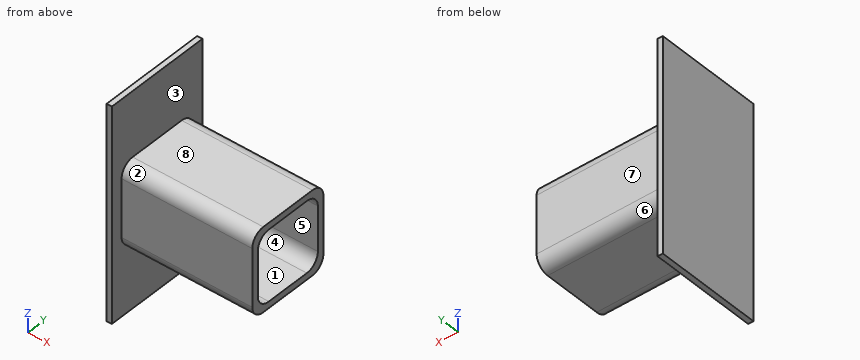
from build123d import *

# Parameters (mm, degrees)
SKETCH1_W           = 164
SKETCH1_H           = 82
BOSS_EXTRUDE1_DEPTH = 4
BOSS_EXTRUDE5_DEPTH = 100


with BuildPart() as part:
    # Sketch1 → Boss-Extrude1 (new body)
    with BuildSketch(Plane(origin=(0, 0, 0), x_dir=(0, 0, -1), z_dir=(1, 0, 0))):
        Rectangle(SKETCH1_W, SKETCH1_H)
    extrude(amount=BOSS_EXTRUDE1_DEPTH)

    # Sketch7 → Boss-Extrude5 (add)
    with BuildSketch(Plane(origin=(4, 0, 0), x_dir=(0, 0, -1), z_dir=(1, 0, 0))):
        with BuildLine():
            Line((-22.18, -32.18), (22.18, -32.18))
            ThreePointArc((22.18, -32.18), (29.251067812, -29.251067812), (32.18, -22.18))
            Line((32.18, -22.18), (32.18, 22.18))
            ThreePointArc((32.18, 22.18), (29.251067812, 29.251067812), (22.18, 32.18))
            Line((22.18, 32.18), (-22.18, 32.18))
            ThreePointArc((-22.18, 32.18), (-29.251067812, 29.251067812), (-32.18, 22.18))
            Line((-32.18, 22.18), (-32.18, -22.18))
            ThreePointArc((-32.18, -22.18), (-29.251067812, -29.251067812), (-22.18, -32.18))
        make_face()
        with BuildLine():
            Line((-17.18, -27.18), (17.18, -27.18))
            ThreePointArc((17.18, -27.18), (24.251067812, -24.251067812), (27.18, -17.18))
            Line((27.18, -17.18), (27.18, 17.18))
            ThreePointArc((27.18, 17.18), (24.251067812, 24.251067812), (17.18, 27.18))
            Line((17.18, 27.18), (-17.18, 27.18))
            ThreePointArc((-17.18, 27.18), (-24.251067812, 24.251067812), (-27.18, 17.18))
            Line((-27.18, 17.18), (-27.18, -17.18))
            ThreePointArc((-27.18, -17.18), (-24.251067812, -24.251067812), (-17.18, -27.18))
        make_face(mode=Mode.SUBTRACT)
    extrude(amount=BOSS_EXTRUDE5_DEPTH)


solid = part.part
For this review, take the finished solid that the model builds, in its own axes (mm). Face numbers are marked on the shaded views. A direction names the side the tool comes from. Give positions to 0.01 mm unless a question says otherwise; leave off trailing zeros. Order: outer loops, then holes, each group sorted by start corner. A loop starts at its lowest first (then second) coordinate and runs counter-clockwise, first axis right, second up. Notation, with made-up numbers: M 1.25,82.5 L 18.25,82.5 A8 cw 18.25,89.5 Z; hole C 64.5,-7 d2. An arc over 180 degrees is marked long. Answer in a Markdown table with one row per item. Add a question column.
(1) Wall thickness on probe 1 along Y at (x, z) = (10, -7.5); probe 2 along X at (y, z) = (14, -73.5): over which ranges is each line inside the solid? List them lowest first. Write a range as [from, to].
(2) Consider section A-A on x = 47. State the section outline as (y, z) points.
(3) For pin 1 (17 mm diameter, centred on x = 49, y = -1, fed in from -Z); pin 2 (17 mm diameter, centred on x = 66.5, y = 8.5, fed in from +Z); pin 3 (5 mm diameter, centred on y = -10.5, z = -2.5, fed in from +X), all flat-tipped, find the tip position at first contact; note any pin that passes through.
(4) Consider section C-C on y = 11.5. State the section outline as (x, z) points.
(5) Mouldability with a two-part tool opening along Y and no side actions: class the marked faces 1, 2, 3 and 4 as +Y half, -Y half, draft (parallel to the pull), parting line (faces both ways), or undercut.
(6) For the marked faces 5, 6, 7 and 8, list the 3-axis set-ups (+Z, -Z, +X, -X, +Y, -Y) from which the entire face can be reached by the end or side of a thin tool; tool diameter is ignored.
(7) Consider section D-D on z = -60. State the section outline as (x, y) points.
(8) Consider section B-B on z = -4. State the section outline as (x, y) points.
Evaluation:
| question | item | result |
|---|---|---|
| 1 | probe 1 | y = [-32.18, -27.18], [27.18, 32.18] |
| 1 | probe 2 | x = [0, 4] |
| 2 | outline | M -32.18,-22.18 A10 ccw -22.18,-32.18 L 22.18,-32.18 A10 ccw 32.18,-22.18 L 32.18,22.18 A10 ccw 22.18,32.18 L -22.18,32.18 A10 ccw -32.18,22.18 Z; hole M -27.18,-17.18 A10 ccw -17.18,-27.18 L 17.18,-27.18 A10 ccw 27.18,-17.18 L 27.18,17.18 A10 ccw 17.18,27.18 L -17.18,27.18 A10 ccw -27.18,17.18 Z |
| 3 | pin 1 | stops at z = -32.18 |
| 3 | pin 2 | stops at z = 32.18 |
| 3 | pin 3 | stops at x = 4 |
| 4 | outline | M 0,-82 L 4,-82 L 4,-32.18 L 104,-32.18 L 104,-27.18 L 4,-27.18 L 4,27.18 L 104,27.18 L 104,32.18 L 4,32.18 L 4,82 L 0,82 Z |
| 5 | face 1 | undercut |
| 5 | face 2 | -Y half |
| 5 | face 3 | draft |
| 5 | face 4 | undercut |
| 6 | face 5 | +X |
| 6 | face 6 | -Z, +X, +Y |
| 6 | face 7 | +Z, -Z, +X, +Y |
| 6 | face 8 | +Z, +X, +Y, -Y |
| 7 | outline | M 0,-41 L 4,-41 L 4,41 L 0,41 Z |
| 8 | outline | M 0,-41 L 4,-41 L 4,-32.18 L 104,-32.18 L 104,-27.18 L 4,-27.18 L 4,27.18 L 104,27.18 L 104,32.18 L 4,32.18 L 4,41 L 0,41 Z |
